from build123d import *

# Parameters (mm, degrees)
SKETCH1_R      = 1.1
BOARD_DEPTH    = 0.8
ESQUISSE1_W    = 14
ESQUISSE1_H    = 20
CAPTEURS_DEPTH = 1


with BuildPart() as part:
    # Sketch1 → Board (new body)
    with BuildSketch(Plane(origin=(0, 0, 0), x_dir=(1, 0, 0), z_dir=(0, 1, 0))):
        with BuildLine():
            Line((0.8, 0), (8, 0))
            ThreePointArc((8, 0), (10, 2), (12, 0))
            Line((12, 0), (19.2, 0))
            ThreePointArc((19.2, 0), (19.765685425, 0.234314575), (20, 0.8))
            Line((20, 0.8), (20, 8))
            ThreePointArc((20, 8), (22, 10), (20, 12))
            Line((20, 12), (20, 28))
            ThreePointArc((20, 28), (18, 30), (20, 32))
            Line((20, 32), (20, 39.2))
            ThreePointArc((20, 39.2), (19.765685425, 39.765685425), (19.2, 40))
            Line((19.2, 40), (12, 40))
            ThreePointArc((12, 40), (10, 42), (8, 40))
            Line((8, 40), (0.8, 40))
            ThreePointArc((0.8, 40), (0.234314575, 39.765685425), (0, 39.2))
            Line((0, 39.2), (0, 32))
            ThreePointArc((0, 32), (2, 30), (0, 28))
            Line((0, 28), (0, 12))
            ThreePointArc((0, 12), (-2, 10), (0, 8))
            Line((0, 8), (0, 0.8))
            ThreePointArc((0, 0.8), (0.234314575, 0.234314575), (0.8, 0))
        make_face()
        with Locations(Location((10, 40, 0), (0, 0, 270))):
            Circle(SKETCH1_R, mode=Mode.SUBTRACT)
        with Locations(Location((0, 10, 0), (0, 0, 270))):
            Circle(SKETCH1_R, mode=Mode.SUBTRACT)
        with Locations(Location((20, 10, 0), (0, 0, 270))):
            Circle(SKETCH1_R, mode=Mode.SUBTRACT)
    extrude(amount=BOARD_DEPTH)

    # Esquisse1 → Capteurs (add)
    with BuildSketch(Plane(origin=(0, 0.8, 0), x_dir=(1, 0, 0), z_dir=(0, 1, 0))):
        with Locations((10, 13)):
            Rectangle(ESQUISSE1_W, ESQUISSE1_H)
    extrude(amount=CAPTEURS_DEPTH)


solid = part.part
Here's how the part is built. I have some questions about the finished solid (model axes, mm). A direction names the side the tool comes from. Give positions to 0.01 mm unless a question says otherwise; leave off trailing zeros. Loops run counter-clockwise (first coordinate to the right, second up) from the corner with the lowest first, then second, coordinate; pieces in that order, holes last. Notation, with made-up numbers: (45, 64.5) -> (100, 64.5) arc R8 cw to (100, 78.5) -> close; hole circle Ø11 at (-24.5, -38.75). An arc over 180 degrees is marked (long way). One line per item, written item: value.
Q1. If I drill on line 1 along X through (y, z) = (0.4, -10); line 2 along X through (y, z) = (1.15, -13); line 3 along Y through (x, z) = (1, -37), over which ranges is the centre line in solid material (lowest first)?
Answers follow:
line 1: -2 to -1.1, 1.1 to 18.9, 21.1 to 22
line 2: 3 to 17
line 3: 0 to 0.8
Q2. Suppose I cut it at B-B on x = 10.5. Please give me the cut outline in (y, z).
Answers follow:
outline: (0, -41.94) -> (0.8, -41.94) -> (0.8, -40.98) -> (0, -40.98) -> close; (0, -39.02) -> (0.8, -39.02) -> (0.8, -23) -> (1.8, -23) -> (1.8, -3) -> (0.8, -3) -> (0.8, -1.94) -> (0, -1.94) -> close
Q3. On a 3-axis mill with a long thin cutter (end or side, diameter ignored), from which of +Z, -Z, +X, -X, +Y, -Y can I reach the whole of each face in a straight line? I mean faces 1 (the face through (10, 1, -23)), 2 (the face through (17, 1, -13)), 3 (the face through (10, 1, -3)), 4 (the face through (-0.421, 0.394, -8.984)), 5 (the face through (10, 0, -21)). Say none if no direction works.
Answers follow:
face 1: -Z, +X, -X, +Y
face 2: +Z, -Z, +X, +Y
face 3: +Z, +X, -X, +Y
face 4: +Y, -Y
face 5: +Z, -Z, +X, -X, -Y
Q4. Suppose I cut it at D-D on z = -25.5. Please give me the cut outline in (x, y), then the cut area to 3 significant figures.
Answers follow:
outline: (0, 0) -> (20, 0) -> (20, 0.8) -> (0, 0.8) -> close
area: 16.0 mm^2
Q5. Suppose I cut it at A-A on z = -10. Please give me the cut outline in (x, y), then the cut area to 3 significant figures.
Answers follow:
outline: (-2, 0) -> (-1.1, 0) -> (-1.1, 0.8) -> (-2, 0.8) -> close; (1.1, 0) -> (18.9, 0) -> (18.9, 0.8) -> (17, 0.8) -> (17, 1.8) -> (3, 1.8) -> (3, 0.8) -> (1.1, 0.8) -> close; (21.1, 0) -> (22, 0) -> (22, 0.8) -> (21.1, 0.8) -> close
area: 29.7 mm^2
Q6. Suppose I cut it at C-C on x = 5.75. Please give me the cut outline in (y, z), then the cut area to 3 significant figures.
Answers follow:
outline: (0, -40) -> (0.8, -40) -> (0.8, -23) -> (1.8, -23) -> (1.8, -3) -> (0.8, -3) -> (0.8, 0) -> (0, 0) -> close
area: 52.0 mm^2
Q7. We'd pull the mould along X, two halves only. Please class faces 6 (the face through (3, 1, -13)), 7 (the face through (10, 0.4, -2)), 8 (the face through (22, 0.4, -10)): pulls with the +X half, pulls with the -X half, needs draft (parallel to the pull), parting line crosses it, or undercut.
Answers follow:
face 6: pulls with the -X half
face 7: undercut
face 8: pulls with the +X half
Q8. I'm going to push flat-ended pins straight in: pin 1 Ø0.6 at (y, z) = (0.5, -36.5) entering from -X; pin 2 Ø0.9 at (y, z) = (0.5, -20) entering from +X; pin 3 Ø3 at (x, z) = (0, -10) entering from +Y; pin 4 Ø1.3 at (x, z) = (20, -10) entering from +Y. Where does each tip first touch, or does it pass through?
Answers follow:
pin 1: x = 0
pin 2: x = 20
pin 3: y = 0.8
pin 4: through
